The drawing under review shows one solid part. Ordinate dimensions are in mm from its lowest x, y, z. Coordinates: 2 decimals unless noted, no trailing zeros. Order: outer loops, then holes, each group sorted by start corner. A loop starts at its lowest first (then second) coordinate and runs counter-clockwise, first axis right, second up.
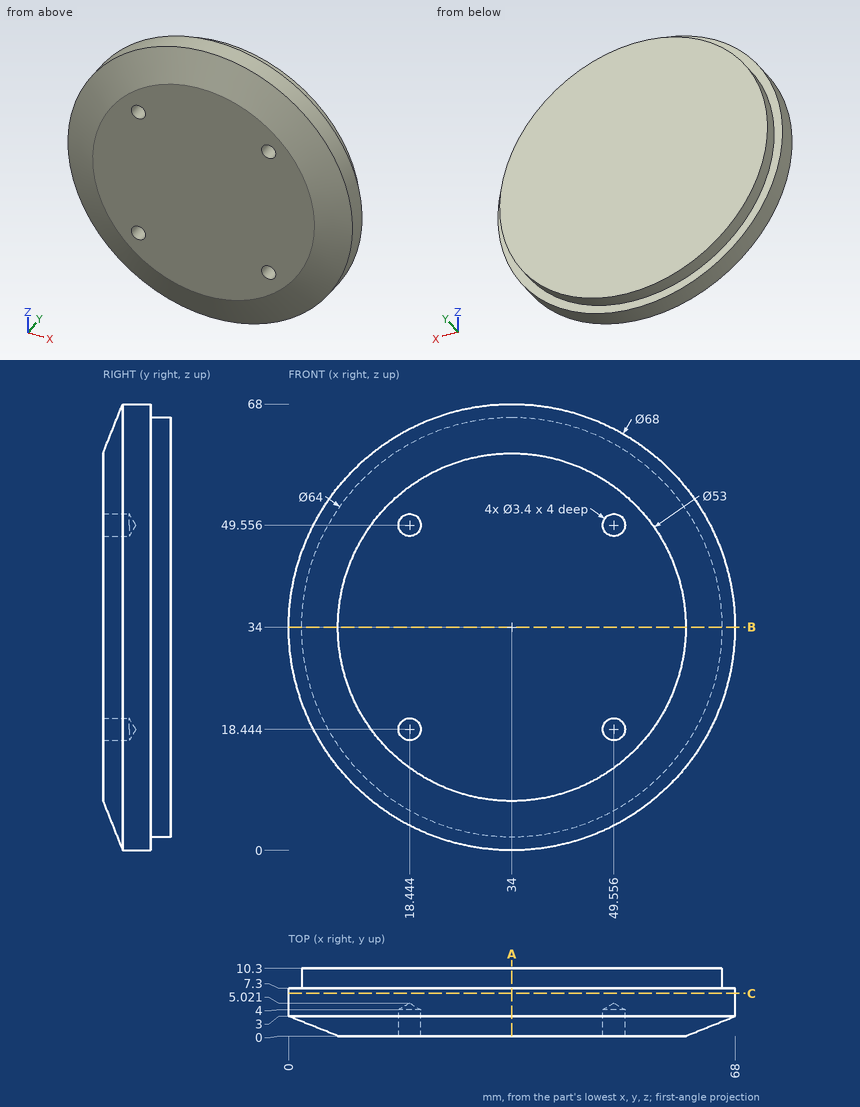
(1) We need section B-B, the plane z = 34. Write out the cut boundary in (x, y).
A:
outline: (0, 3) - (7.5, 0) - (60.5, 0) - (68, 3) - (68, 7.3) - (66, 7.3) - (66, 10.3) - (2, 10.3) - (2, 7.3) - (0, 7.3) - close
(2) For pin 1 Ø4 at (x, z) = (12, 56) entering from -Y (1 decimal); pin 2 Ø1.5 at (x, y) = (38, 4) entering from +Z; pin 3 Ø4 at (x, y) = (53, 1.5) entering from +Z (1 decimal), all flat-tipped, find the tip position at first contact; note any pin that passes through.
A:
pin 1: stops at y = 1
pin 2: stops at z = 67.84
pin 3: stops at z = 63
(3) We need section C-C, the plane y = 6.5. Write out the cut boundary in (x, z).
A:
outline: circle Ø68 at (34, 34)
(4) Wall thickness on probe 1 along Z at (x, y) = (18.5, 3.75) (1 decimal); probe 2 along Z at (x, y) = (46, 8) (1 decimal); probe 3 along X at (y, z) = (6.25, 8): over which ranges is each line inside the solid? List them lowest first.
A:
probe 1: z = 3.7 to 16.7, 20.1 to 47.9, 51.3 to 64.3
probe 2: z = 4.3 to 63.7
probe 3: x = 12.09 to 55.91
(5) We need section A-A, the plane x = 34. Write out the cut boundary in (y, z), and give its area (3 significant figures).
A:
outline: (0, 7.5) - (3, 0) - (7.3, 0) - (7.3, 2) - (10.3, 2) - (10.3, 66) - (7.3, 66) - (7.3, 68) - (3, 68) - (0, 60.5) - close
area: 666 mm2
